The model under review builds one solid part; all positions refer to its coordinate system, in mm. Face numbers are marked on the shaded views. A direction names the side the tool comes from. Give positions to 0.01 mm unless a question says otherwise; leave off trailing zeros. Order: outer loops, then holes, each group sorted by start corner. A loop starts at its lowest first (then second) coordinate and runs counter-clockwise, first axis right, second up. Notation, with made-up numbers: (47.5, 17) - (92.5, 17) arc R29 cw to (92.5, 40) - close; hole circle Ø7 at (-3.5, -32). An arc over 180 degrees is marked (long way). Write item = value, one per line. Start each with the question number.
1. For P1, Ø4, axis at x = 22, y = 10.5, coming from the +Z side, flat-tipped, find the tip position at first contact; note if it passes through.
2. We need section C-C, the plane x = 36. Give the boundary of the cut face in (y, z).
3. We need section B-B, the plane x = 19. Give the boundary of the cut face in (y, z), and give its area (3 significant figures).
4. We need section D-D, the plane z = 11. Give the boundary of the cut face in (x, y).
5. Machinability: for the marked faces 1 and 2, which of the approach directions +Z, -Z, +X, -X, +Y, -Y give a long, thin tool a straight path to every point of the face, cutting with its end or side? Answer none if there is none.
6. We need section A-A, the plane z = 31. Give the boundary of the cut face in (x, y).
7. Wall thickness on probe 1 along Z at (x, y) = (12, 22.75): over which ranges is the line inside the solid? List them lowest first.
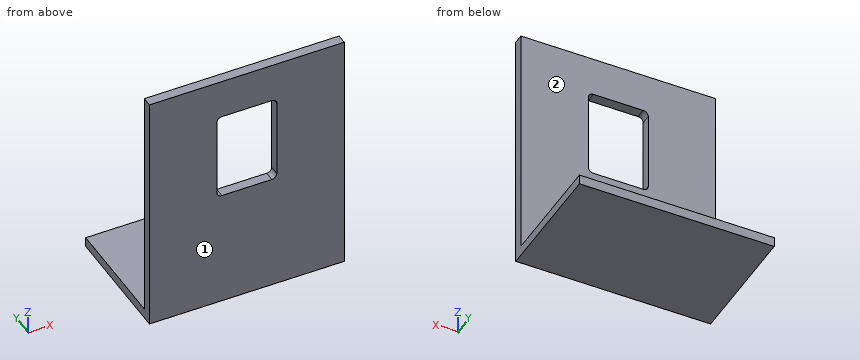
Autodesk Inventor part; units mm, degrees
ref_plane "YZ Plane" through (0, 0, 0) normal (1, 0, 0) x (0, 1, 0)
ref_plane "XZ Plane" through (0, 0, 0) normal (0, 1, 0) x (-1, 0, 0)
ref_plane "XY Plane" through (0, 0, 0) normal (0, 0, 1) x (1, 0, 0)
sketch "Sketch1" plane through (0, 0, 0) normal (0, 0, 1) x (1, 0, 0)
  line L0 (0, 0) -> (39, 0)
  line L1 (39, 0) -> (39, 24.8)
  line L2 (39, 24.8) -> (0, 24.8)
  line L3 (0, 24.8) -> (0, 0)
  dimension "d0" = 39
  dimension "d1" = 24.8
extrude "Extrusion1" add sketch "Sketch1" along normal blind 2
sketch "Sketch2" plane through (0, 0, 2) normal (0, 0, 1) x (1, 0, 0)
  line L0 (0, 24.8) -> (0, 0)
  line L1 (0, 0) -> (39, 0)
  line L2 (39, 0) -> (39, 2)
  line L3 (39, 2) -> (0, 2)
  line L4 (0, 2) -> (0, 0)
  dimension "d4" = 39
  dimension "d5" = 2
extrude "Extrusion2" add sketch "Sketch2" along normal blind 48
sketch "Sketch3" plane through (0, 0, 0) normal (0, -1, 0) x (1, 0, 0)
  line L0 (0, 0) -> (39, 0)
  line L1 (19.5, 24) -> (24.5, 24)
  line L2 (25.5, 25) -> (25.5, 41)
  line L3 (24.5, 42) -> (14.5, 42)
  line L4 (13.5, 41) -> (13.5, 25)
  line L5 (14.5, 24) -> (19.5, 24)
  arc A0 (14.5, 42) -> (13.5, 41) centre (14.5, 41) ccw
  arc A1 (24.5, 24) -> (25.5, 25) centre (24.5, 25) ccw
  arc A2 (25.5, 41) -> (24.5, 42) centre (24.5, 41) ccw
  arc A3 (13.5, 25) -> (14.5, 24) centre (14.5, 25) ccw
  point P0 (25.5, 24)
  point P1 (25.5, 42)
  point P2 (13.5, 42)
  point P3 (13.5, 24)
  dimension "d9" = 6
  dimension "d10" = 18
  dimension "d11" = 12
  dimension "d12" = 18
  dimension "d13" = 1
extrude "Extrusion3" cut sketch "Sketch3" against normal blind 48
properties part number "Kamera 2"
Model answer:
q1.P1 = 2
q2.outline = (0, 0) - (24.8, 0) - (24.8, 2) - (2, 2) - (2, 50) - (0, 50) - close
q3.outline = (0, 0) - (24.8, 0) - (24.8, 2) - (2, 2) - (2, 24) - (0, 24) - close; (0, 42) - (2, 42) - (2, 50) - (0, 50) - close
q3.area = 110 mm2
q4.outline = (0, 0) - (39, 0) - (39, 2) - (0, 2) - close
q5.face_1 = +Z, -Z, +X, -X, -Y
q5.face_2 = +Z, +X, -X, +Y
q6.outline = (0, 0) - (13.5, 0) - (13.5, 2) - (0, 2) - close; (25.5, 0) - (39, 0) - (39, 2) - (25.5, 2) - close
q7.probe_1 = 0 to 2
